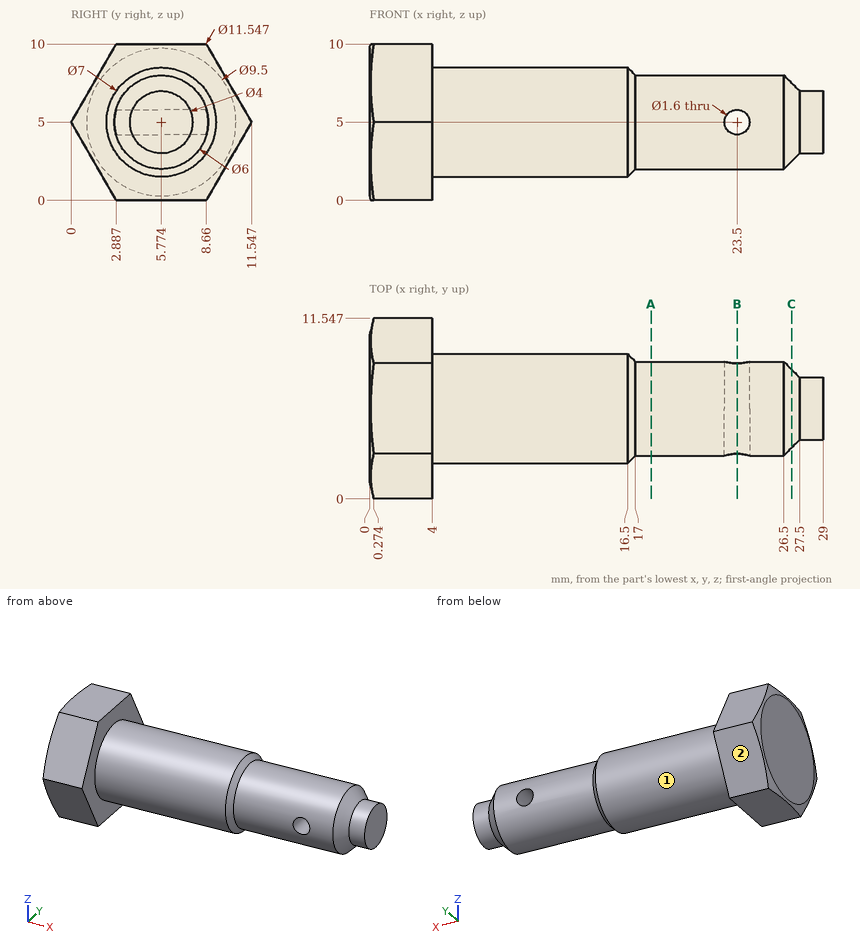
The figure shows three views and two pictorial views of one solid part (mm, origin at its lowest corner). Answer the questions. A direction names the side the tool comes from. Give positions to 0.01 mm unless a question says otherwise; leave off trailing zeros. Loops run counter-clockwise (first coordinate to the right, second up) from the corner with the lowest first, then second, coordinate; pieces in that order, holes last. Notation, with made-up numbers: (14.25, 56.25) -> (39.25, 56.25) arc R21 ccw to (39.25, 78.25) -> close; hole circle Ø3 at (-9.5, -20.75). An arc over 180 degrees is marked (long way). Put each result on its own line as item: value. Start each with the question number.
Item 1: The part is cut by section B-B (x = 23.5). Give the vertices of the cut face in (y, z) (1 decimal).
Item 2: Which of the six approach directions +Z, -Z, +X, -X, +Y, -Y give full straight-line access (tool end or side, diameter ignored) to the marked faces 1 and 2?
Item 3: Each of these flat-tipped pins is pushed along its axis until it touches: P1, Ø5, axis at x = 4.5, z = 3, coming from the +Y side; P2, Ø1.8, axis at x = 23.5, z = 5, coming from the -Y side; P3, Ø3, axis at x = 6.5, y = 5, coming from the -Z side; P4, Ø2, axis at x = 13, z = 3, coming from the -Y side. Where does it stop, or does it pass through?
Item 4: Find the intervals of material crossed by L1, parallel to X at y = 8, z = 1.5; L2, parallel to Z at x = 23.5, y = 6.45; L3, parallel to X at y = 1.25, z = 7, in increasing order. Write a range as [from, to].
Item 5: The part is cut by section A-A (x = 18). Give the vertices of the cut face in (y, z).
Item 6: The part is cut by section C-C (x = 27). Give the vertices of the cut face in (y, z).
Answers below:
1. outline: (2.9, 4.2) arc R3 ccw to (8.7, 4.2) -> close; (2.9, 5.8) -> (8.7, 5.8) arc R3 ccw to start
2. face 1: +X
2. face 2: -Z, +X, -X, +Y
3. P1: y = 11.55
3. P2: y = 2.77
3. P3: z = 1.5
3. P4: y = 2.42
4. L1: [0, 4]
4. L2: [2.08, 4.2], [5.8, 7.92]
4. L3: [0.05, 4]
5. outline: circle Ø6 at (5.77, 5)
6. outline: circle Ø5 at (5.77, 5)
